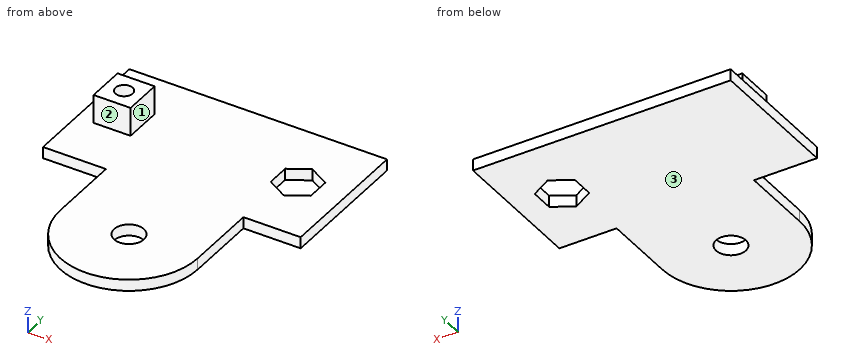
from build123d import *

# Parameters (mm, degrees)
F1_DEPTH = 2
F2_W     = 6.4592821483
F2_H     = 6.7308258385
F2_R     = 1.5
F3_DEPTH = 5
F4_R     = 1.5
F5_DEPTH = 2


with BuildPart() as f1:
    # F0 (on Top) → F1 (new body)
    with BuildSketch(Plane.XY):
        Polygon((19.8, 29.7919024055), (-25.2, 29.7919024055), (-25.2, 5.5919024055), (-14.2, 5.5919024055), (9.8, 5.5919024055), (19.8, 5.5919024055), align=None)
        with BuildLine():
            Line((9.8, 5.5919024055), (-14.2, 5.5919024055))
            Line((-14.2, 5.5919024055), (-14.2, -7.2080975945))
            Line((-14.2, -7.2080975945), (-4.8, -7.2080975945))
            ThreePointArc((-4.8, -7.2080975945), (-2.2, -4.6080975945), (0.4, -7.2080975945))
            Line((0.4, -7.2080975945), (9.8, -7.2080975945))
            Line((9.8, -7.2080975945), (9.8, 5.5919024055))
        make_face()
        with BuildLine():
            Line((-4.8, -7.2080975945), (-14.2, -7.2080975945))
            ThreePointArc((-14.2, -7.2080975945), (-2.2, -19.2080975945), (9.8, -7.2080975945))
            Line((9.8, -7.2080975945), (0.4, -7.2080975945))
            ThreePointArc((0.4, -7.2080975945), (-2.2, -9.8080975945), (-4.8, -7.2080975945))
        make_face()
    extrude(amount=F1_DEPTH)

    # F2 (on face) → F3 (join)
    with BuildSketch(Plane.XY.offset(2)):
        with Locations((-18.9703589258, 18.3236696757)):
            Rectangle(F2_W, F2_H)
        with Locations((-18.9703589258, 18.3236696757)):
            Circle(F2_R, mode=Mode.SUBTRACT)
    extrude(amount=F3_DEPTH)

    # F4 (on face) → F5 (cut, through all)
    with BuildSketch(Plane.XY.offset(2)):
        Polygon((15.3, 15.6711764633), (15.3, 19.7126283476), (11.8, 21.7333542898), (8.3, 19.7126283476), (8.3, 15.6711764633), (11.8, 13.6504505211), align=None)
        with Locations((11.8, 17.6919024055)):
            Circle(F4_R, mode=Mode.SUBTRACT)
        with Locations((11.8, 17.6919024055)):
            Circle(F4_R)
    extrude(amount=-F5_DEPTH, mode=Mode.SUBTRACT)


solid = f1.part
Geometry check sheet. Reference: the model listing, model coordinates, mm. Face numbers are marked on the shaded views. A direction names the side the tool comes from. Give positions to 0.01 mm unless a question says otherwise; leave off trailing zeros. Write each loop counter-clockwise with the first axis right and the second up, starting at its lowest first coordinate (ties: lowest second). Pieces come first, ordered by that corner, then holes.
1) Thickness scan on line 1 (Y direction, x = -2.2, z = 0.8); line 2 (X direction, y = -9, z = 1.5); line 3 (X direction, y = 19.5, z = 2.5). Record the ranges inside material, lowest first.
Values follow:
line 1: y = -19.21 to -9.81, -4.61 to 29.79
line 2: x = -14.07 to -4.08, -0.32 to 9.67
line 3: x = -22.2 to -19.9, -18.04 to -15.74
2) Cross-section at D-D (x = 11). Record the boundary of the cut face in (y, z), plus the area to 3 significant figures.
Values follow:
outline: (5.59, 0) - (14.11, 0) - (14.11, 2) - (5.59, 2) - close; (21.27, 0) - (29.79, 0) - (29.79, 2) - (21.27, 2) - close
area: 34.1 mm2
3) Cross-section at A-A (x = -2.2). Record the boundary of the cut face in (y, z), plus the area to 3 significant figures.
Values follow:
outline: (-19.21, 0) - (-9.81, 0) - (-9.81, 2) - (-19.21, 2) - close; (-4.61, 0) - (29.79, 0) - (29.79, 2) - (-4.61, 2) - close
area: 87.6 mm2
4) Set-up check for the marked faces 1, 2 and 3: record each of +Z, -Z, +X, -X, +Y, -Y from which the full face is reachable in a straight line by a thin tool's end or side.
Values follow:
face 1: +Z, +X, +Y, -Y
face 2: +Z, +X, -X, -Y
face 3: -Z, +X, -X, +Y, -Y
5) Go/stop test with flat-tipped pins: pin 1 Ø12 at (x, y) = (2, 8.5) entering from +Z; pin 2 Ø1.5 at (y, z) = (17, 3.5) entering from +X; pin 3 Ø0.6 at (y, z) = (1.5, 0.5) entering from -X. Record where each tip stops, or that it passes through.
Values follow:
pin 1: stops at z = 2
pin 2: stops at x = -15.74
pin 3: stops at x = -14.2
6) Cross-section at C-C (y = 22.5). Record the boundary of the cut face in (x, z), plus the area to 3 significant figures.
Values follow:
outline: (-25.2, 0) - (19.8, 0) - (19.8, 2) - (-25.2, 2) - close
area: 90.0 mm2
7) Cross-section at B-B (z = 6). Record the boundary of the cut face in (x, y), plus the area to 3 significant figures.
Values follow:
outline: (-22.2, 14.96) - (-15.74, 14.96) - (-15.74, 21.69) - (-22.2, 21.69) - close; hole circle Ø3 at (-18.97, 18.32)
area: 36.4 mm2
